Verification items for the finished model (mm, model axes). Coordinates: 2 decimals unless noted, no trailing zeros. Write each loop counter-clockwise with the first axis right and the second up, starting at its lowest first coordinate (ties: lowest second). Pieces come first, ordered by that corner, then holes. Notation, with made-up numbers: (59, -7.5) -> (116, -7.5) arc R15 cw to (116, 15.5) -> close; hole circle Ø8 at (5.25, 60). An arc over 180 degrees is marked (long way). Use CSV: the item, a comma, the result in double quotes.
Solid Edge part; units mm, degrees
sketch "Sketch1" plane through (0, 0, 0) normal (0, 0, 1) x (1, 0, 0)
  line L0 (-15.75, -20) -> (15.75, -20)
  line L1 (15.75, -20) -> (15.75, 20)
  line L2 (15.75, 20) -> (-15.75, 20)
  line L3 (-15.75, 20) -> (-15.75, -20)
  dimension "D1" = 15.75
  dimension "D2" = 15.75
extrude "Protrusion1" add sketch "Sketch1" along normal mid plane 1
sketch "Sketch2" plane through (0, 0, 0.5) normal (0, 0, 1) x (1, 0, 0)
  circle A0 centre (0, 10) radius 2.25
  circle A1 centre (0, -10) radius 2.25
extrude "Cutout1" cut sketch "Sketch2" against normal through all
chamfer "Chamfer_1" distance 0.5 angle 45 2 edges at (-2.25, 10, 0.5) (-2.25, -10, 0.5)
properties material "Polyethylene, low density"
1) Mould release check, pull along X, two halves, no side actions. Record for faces 1 (the flat face through (-15.75, 0, 0)), 2 (the cylindrical face through (-0.29, -7.77, -0.25)), 3 (the cylindrical face through (1.21, 11.897, -0.246)), 4 (the flat face through (0, -20, 0)): released by +X, released by -X, zero draft, split by the parting line, or undercut.
Return value:
face 1,"released by -X"
face 2,"undercut"
face 3,"undercut"
face 4,"zero draft"
2) Cross-section at B-B (z = 0.2). Record the boundary of the cut face in (x, y), plus the area to 3 significant figures.
Return value:
outline,"(-15.75, -20) -> (15.75, -20) -> (15.75, 20) -> (-15.75, 20) -> close; hole circle Ø4.9 at (0, -10); hole circle Ø4.9 at (0, 10)"
area,"1,220 mm2"
3) Cross-section at A-A (x = 0). Record the boundary of the cut face in (y, z).
Return value:
outline,"(-20, -0.5) -> (-12.25, -0.5) -> (-12.25, 0) -> (-12.75, 0.5) -> (-20, 0.5) -> close; (-7.75, -0.5) -> (7.75, -0.5) -> (7.75, 0) -> (7.25, 0.5) -> (-7.25, 0.5) -> (-7.75, 0) -> close; (12.25, -0.5) -> (20, -0.5) -> (20, 0.5) -> (12.75, 0.5) -> (12.25, 0) -> close"
4) Cross-section at C-C (y = -10). Record the boundary of the cut face in (x, z), plus the area to 4 significant figures.
Return value:
outline,"(-15.75, -0.5) -> (-2.25, -0.5) -> (-2.25, 0) -> (-2.75, 0.5) -> (-15.75, 0.5) -> close; (2.25, -0.5) -> (15.75, -0.5) -> (15.75, 0.5) -> (2.75, 0.5) -> (2.25, 0) -> close"
area,"26.75 mm2"
5) Scan lines: L1, parallel to Y at x = 0, z = -0.2; L2, parallel to Y at x = 1.5, z = 0.35; L3, parallel to X at y = -9, z = 0. Record each from-to range of solid material in increasing order.
Return value:
L1,"-20 to -12.25, -7.75 to 7.75, 12.25 to 20"
L2,"-20 to -12.12, -7.88 to 7.88, 12.12 to 20"
L3,"-15.75 to -2.02, 2.02 to 15.75"
